Here's how the part is built. I have some questions about the finished solid (model axes, mm). A direction names the side the tool comes from. Round coordinates to 2 decimals unless told otherwise and drop trailing zeros. Loops run counter-clockwise (first coordinate to the right, second up) from the corner with the lowest first, then second, coordinate; pieces in that order, holes last. Notation, with made-up numbers: M 46,-17.75 L 100,-17.75 A15 ccw 100,-9.75 Z; hole C -26,-3.75 d6. An arc over 180 degrees is marked long. Answer as a JSON object with one key per item and string values.
from build123d import *

# Parameters (mm, degrees)
REVOLVE2_ANGLE      = 90
SKETCH3_W           = 3
SKETCH3_H           = 12
BOSS_EXTRUDE1_DEPTH = 3


with BuildPart() as part:
    # Sketch1 → Revolve2 (revolve)
    with BuildSketch(Plane.XY):
        with BuildLine():
            Line((-55.793660937, -33.37535625), (-63.601425001, -2.144299994))
            Line((-63.601425001, -2.144299994), (-63.9, 0.281056256))
            Line((-63.9, 0.281056256), (-63.9, 30.95))
            ThreePointArc((-63.9, 30.95), (-60.971067812, 38.021067812), (-53.9, 40.95))
            Line((-53.9, 40.95), (-43.9, 40.95))
            Line((-43.9, 40.95), (-43.9, 37.95))
            Line((-43.9, 37.95), (-53.9, 37.95))
            ThreePointArc((-53.9, 37.95), (-58.849747468, 35.899747468), (-60.9, 30.95))
            Line((-60.9, 30.95), (-60.9, 0.281056256))
            Line((-60.9, 0.281056256), (-60.690997501, -1.416693119))
            Line((-60.690997501, -1.416693119), (-55.793660937, -21.006039374))
            Line((-55.793660937, -21.006039374), (-52.883233437, -32.647749375))
            ThreePointArc((-52.883233437, -32.647749375), (-50.400121402, -36.467438066), (-46.092235936, -37.95))
            Line((-46.092235936, -37.95), (-43.9, -37.95))
            Line((-43.9, -37.95), (-43.9, -40.95))
            Line((-43.9, -40.95), (-46.092235936, -40.95))
            ThreePointArc((-46.092235936, -40.95), (-52.24635803, -38.83205438), (-55.793660937, -33.37535625))
        make_face()
    revolve(axis=Axis((-43.9, 40.95, 0), (0, 1, 0)), revolution_arc=REVOLVE2_ANGLE)

    # Sketch3 → Boss-Extrude1 (add)
    with BuildSketch(Plane(origin=(0, 0, 0), x_dir=(-1, 0, 0), z_dir=(0, 0, -1))):
        Polygon((55.793660937, -33.37535625), (58.711666985, -21.70333206), (55.793660937, -21.006039374), (52.883233437, -32.647749375), align=None)
        with Locations((62.4, 24.95)):
            Rectangle(SKETCH3_W, SKETCH3_H)
    extrude(amount=BOSS_EXTRUDE1_DEPTH)


solid = part.part
Item 1: For faces 4 (the face through (-60.9, 25, -1)), 5 (the face through (-53.8, 38.2, 0)), 6 (the face through (-54.3, -33, -1.5)), which set-ups out of +Z, -Z, +X, -X, +Y, -Y let a thin tool reach every point of the face, with its end or its side?
Solution:
{"face 4": "-Z, +X, +Y, -Y", "face 5": "-Z, +X, -X, +Y", "face 6": "-Z, +X, -Y"}
Item 2: For P1, Ø1, axis at x = -60.5, y = 28, coming from the +Z side; P2, Ø10, axis at x = -60, y = -30.5, coming from the -Z side; P3, Ø4, axis at x = -54, y = 27, coming from the +Z side; P4, Ø3.5, axis at y = 28, z = -1, coming from the +X side, each with a flat end and sliding along its axis, tell me the tip position at first contact or that it passes through.
Solution:
{"P1": "stops at z = 11.87", "P2": "stops at z = -3", "P3": "stops at z = 18.29", "P4": "stops at x = -60.88"}
Item 3: We'd pull the mould along Y, two halves only. Please class faces 1 (the face through (-55.96, -0.77, 11.8)), 2 (the face through (-45, -40.95, 1)), 3 (the face through (-62, 25, -3)): +Y half, -Y half, draft (parallel to the pull), parting line (faces both ways), or undercut.
Solution:
{"face 1": "undercut", "face 2": "-Y half", "face 3": "draft"}
Item 4: If I drill on L1, parallel to Y at x = -48.75, z = 7.25; L2, parallel to Y at x = -50.25, z = 5.5; L3, parallel to Z at x = -51, y = -21, over which ranges is the centre line in solid material (lowest first)? Write a range as from..to.
Solution:
{"L1": "y = -38.52..-33.47, 37.95..40.95", "L2": "y = -38.79..-34.18, 37.95..40.95", "L3": "z = 9.54..13.2"}
Item 5: I want a section at B-B on y = -30.5. List the corners of the cut face in (x, z) for me (1 decimal).
Solution:
{"outline": "M -56.5,-3 L -53.4,-3 L -53.4,0 A9.5 cw -43.9,9.5 L -43.9,12.6 A12.6 ccw -56.5,0 Z"}
Item 6: I want a section at C-C on y = -13. List the corners of the cut face in (x, z) for me (1 decimal).
Solution:
{"outline": "M -60.9,0 L -57.8,0 A13.9 cw -43.9,13.9 L -43.9,17 A17 ccw Z"}
Item 7: I want a section at A-A on y = 5. List the corners of the cut face in (x, z) for me.
Solution:
{"outline": "M -63.9,0 L -60.9,0 A17 cw -43.9,17 L -43.9,20 A20 ccw Z"}
